Geometry: final body of the model. Coordinates: model frame, mm. A direction names the side the tool comes from. Give positions to 0.01 mm unless a question says otherwise; leave off trailing zeros. Loops run counter-clockwise (first coordinate to the right, second up) from the corner with the lowest first, then second, coordinate; pieces in that order, holes last. Notation, with made-up numbers: (-28.75, -37) - (18.25, -37) arc R31 cw to (18.25, -9) - close; hole circle Ø3 at (38, -21.75). An arc over 180 degrees is marked (long way). Answer in a Markdown table with one row per item.
Autodesk Inventor part; units mm, degrees
ref_plane "YZ Plane" through (0, 0, 0) normal (1, 0, 0) x (0, 1, 0)
ref_plane "XZ Plane" through (0, 0, 0) normal (0, 1, 0) x (-1, 0, 0)
ref_plane "XY Plane" through (0, 0, 0) normal (0, 0, 1) x (1, 0, 0)
sketch "Sketch1" plane through (0, 0, 0) normal (0, 0, 1) x (1, 0, 0)
  line L0 (0, 0) -> (3.2004, 0)
  line L1 (3.2004, 0) -> (3.2004, 228.6)
  line L2 (3.2004, 228.6) -> (0, 228.6)
  line L3 (0, 228.6) -> (0, 0)
  dimension "d0" = 3.2004
  dimension "d1" = 228.6
extrude "Extrusion1" add sketch "Sketch1" along normal blind 57.404
sketch "Sketch2" plane through (3.2004, 0, 0) normal (1, 0, 0) x (0, 0, -1)
  line L0 (0, 0) -> (-57.404, 0)
  line L1 (0, 228.6) -> (-57.404, 228.6)
  line L2 (-35.9664, 0) -> (-30.3276, 0)
  line L3 (-30.3276, 0) -> (-30.3276, 228.6)
  line L4 (-30.3276, 228.6) -> (-35.9664, 228.6)
  line L5 (-35.9664, 228.6) -> (-35.9664, 0)
  line L6 (-57.404, 0) -> (-57.404, 228.6)
  dimension "d4" = 228.6
  dimension "d5" = 5.6388
  dimension "d6" = 21.4376
extrude "Extrusion2" add sketch "Sketch2" along normal blind 47.879 contours L0 L5 L1 L3
properties part number "Guide 2"
Q1. Cut plane A-A (y = 63). Output: boundary loops of the cut face in (x, z).
Check values:
| item | result |
|---|---|
| outline | (0, 0) - (3.2, 0) - (3.2, 30.33) - (51.08, 30.33) - (51.08, 35.97) - (3.2, 35.97) - (3.2, 57.4) - (0, 57.4) - close |
Q2. Cut plane C-C (x = 19.5). Output: boundary loops of the cut face in (y, z), and give its area (3 significant figures).
Check values:
| item | result |
|---|---|
| outline | (0, 30.33) - (228.6, 30.33) - (228.6, 35.97) - (0, 35.97) - close |
| area | 1,290 mm² |
Q3. First-contact query: pin 1 (14.5 mm diameter, centred on x = 31.5, y = 163.5, fed in from +Z); pin 2 (24.5 mm diameter, centred on y = 151.5, z = 10.5, fed in from +X); pin 3 (3 mm diameter, centred on y = 191, z = 31, fed in from -X); pin 4 (4 mm diameter, centred on x = 33.5, y = 149.5, fed in from -Z). Flat tips, straight axial feed; report the tip coordinate or a pass-through.
Check values:
| item | result |
|---|---|
| pin 1 | z = 35.97 |
| pin 2 | x = 3.2 |
| pin 3 | x = 0 |
| pin 4 | z = 30.33 |
Q4. Reachability of faces 1 (the flat face through (3.2, 113, 15)), 2 (the flat face through (3.2, 113, 47)), 3 (the flat face through (0, 116, 28)) from +Z, -Z, +X, -X, +Y, -Y: full face, straight path, thin tool, end or side. Return the list, or none.
Check values:
| item | result |
|---|---|
| face 1 | -Z, +X, +Y, -Y |
| face 2 | +Z, +X, +Y, -Y |
| face 3 | +Z, -Z, -X, +Y, -Y |
Q5. Material intervals for line 1 along X through (y, z) = (214, 17); line 2 along Z through (x, y) = (17.5, 84.5), sorted ascending.
Check values:
| item | result |
|---|---|
| line 1 | 0 to 3.2 |
| line 2 | 30.33 to 35.97 |
Q6. Cut plane B-B (z = 10.5). Output: boundary loops of the cut face in (x, y).
Check values:
| item | result |
|---|---|
| outline | (0, 0) - (3.2, 0) - (3.2, 228.6) - (0, 228.6) - close |
